Read the model definition and answer for the solid it produces. Units are mm, in the model's axes. A direction names the side the tool comes from. Coordinates: 2 decimals unless noted, no trailing zeros. Order: outer loops, then holes, each group sorted by start corner. A loop starts at its lowest first (then second) coordinate and runs counter-clockwise, first axis right, second up. Notation, with made-up numbers: M -21.5,24.25 L -8.5,24.25 A27 cw -8.5,55.25 Z; hole C -19,88 d6. An arc over 180 degrees is marked long. Use a Markdown table: item, result. Add a question column.
1) The mould has two halves that part along Z. Classify faces 1 (the face through (5, -493, 49)), 2 (the face through (49, -493, 100)), 3 (the face through (49, -493, 0)), 4 (the face through (46, -1000, 2)): released by +Z, released by -Z, zero draft, split by the parting line, or undercut.
2) For faces 5 (the face through (100, -493, 49)), 6 (the face through (49, -493, 5)), determine the directions among +Z, -Z, +X, -X, +Y, -Y from which every point of the face is accessible in a straight line to the end or side of a thin tool.
3) Find section C-C on y = -718.5. Write down the section's boundary in (x, z).
4) Find section B-B on z = 33. Write down the section's boundary in (x, y), plus the area to 3 significant figures.
5) Find section D-D on z = 85. Write down the section's boundary in (x, y).
6) Find the intervals of material crossed by probe 1 along X at (y, z) = (-123, 97.55); probe 2 along Y at (x, z) = (50, 96); probe 3 along Z at (x, y) = (51, -841), in increasing order. Write a range as [from, to].
7) Find section A-A on x = 72.5. Write down the section's boundary in (y, z).
from build123d import *

# Parameters (mm, degrees)
F0_W     = 100
F0_H     = 100
F0_W_2   = 90
F0_H_2   = 90
F1_DEPTH = 1000
F2_W     = 40
F2_H     = 30
F3_DEPTH = 5
F4_W     = 40
F4_H     = 30
F5_DEPTH = 5
F7_D     = 8.8
F7_DEPTH = 5
F7_TIP   = 2.6437867237


with BuildPart() as f1:
    # F0 (on Front) → F1 (new body)
    with BuildSketch(Plane.XZ):
        with Locations((50, 50)):
            Rectangle(F0_W, F0_H)
        with Locations((50, 50)):
            Rectangle(F0_W_2, F0_H_2, mode=Mode.SUBTRACT)
    extrude(amount=F1_DEPTH)

    # F2 (on face) → F3 (cut)
    with BuildSketch(Plane.YZ.offset(100)):
        with Locations((-887, 79)):
            Rectangle(F2_W, F2_H)
    extrude(amount=-F3_DEPTH, mode=Mode.SUBTRACT)

    # F4 (on face) → F5 (cut)
    with BuildSketch(Plane(origin=(0, 0, 0), x_dir=(0, -1, 0), z_dir=(-1, 0, 0))):
        with Locations((113, 79)):
            Rectangle(F4_W, F4_H)
    extrude(amount=-F5_DEPTH, mode=Mode.SUBTRACT)

    # F7
    with Locations(Plane.XY.offset(100)):
        with Locations((50, -103), (40, -123), (60, -123), (40, -877), (60, -877), (50, -897)):
            Hole(F7_D / 2, depth=F7_DEPTH)
            with Locations((0, 0, -(F7_DEPTH + F7_TIP / 2))):  # 118° drill point
                Cone(0, F7_D / 2, F7_TIP, mode=Mode.SUBTRACT)


solid = f1.part
Check result:
| question | item | result |
|---|---|---|
| 1 | face 1 | undercut |
| 1 | face 2 | released by +Z |
| 1 | face 3 | released by -Z |
| 1 | face 4 | zero draft |
| 2 | face 5 | +Z, -Z, +X, +Y, -Y |
| 2 | face 6 | +Y, -Y |
| 3 | outline | M 0,0 L 100,0 L 100,100 L 0,100 Z; hole M 5,5 L 95,5 L 95,95 L 5,95 Z |
| 4 | outline | M 0,-1000 L 5,-1000 L 5,0 L 0,0 Z; M 95,-1000 L 100,-1000 L 100,0 L 95,0 Z |
| 4 | area | 10,000 mm2 |
| 5 | outline | M 0,-1000 L 5,-1000 L 5,-133 L 0,-133 Z; M 0,-93 L 5,-93 L 5,0 L 0,0 Z; M 95,-1000 L 100,-1000 L 100,-907 L 95,-907 Z; M 95,-867 L 100,-867 L 100,0 L 95,0 Z |
| 6 | probe 1 | x = [0, 35.6], [44.4, 55.6], [64.4, 100] |
| 6 | probe 2 | y = [-1000, -901.4], [-892.6, -107.4], [-98.6, 0] |
| 6 | probe 3 | z = [0, 5], [95, 100] |
| 7 | outline | M -1000,0 L 0,0 L 0,5 L -1000,5 Z; M -1000,95 L 0,95 L 0,100 L -1000,100 Z |
